from build123d import *

# Parameters (mm, degrees)
F1_DEPTH = 50
F3_DEPTH = 25
F4_R     = 9
F5_DEPTH = 25


with BuildPart() as f1:
    # F0 (on Front) → F1 (new body)
    with BuildSketch(Plane.XZ):
        Polygon((48.981464, 6), (-26.018536, 6), (-26.018536, 29), (-36.018536, 29), (-36.018536, -6), (33.685692, -6), (33.685692, -16.768231), (43.685692, -16.768231), (48.981464, -6), align=None)
    extrude(amount=F1_DEPTH)

    # F2 (on face) → F3 (cut)
    with BuildSketch(Plane.YZ.offset(-26.018536)):
        Polygon((-20.902064, 29), (-30.902064, 29), (-30.902064, 21), (-35.902064, 21), (-35.902064, 13), (-15.902064, 13), (-15.902064, 21), (-20.902064, 21), align=None)
    extrude(amount=-F3_DEPTH, mode=Mode.SUBTRACT)

    # F4 (on face) → F5 (cut)
    with BuildSketch(Plane.XY.offset(6)):
        with Locations((13.981464, -25)):
            Circle(F4_R)
    extrude(amount=-F5_DEPTH, mode=Mode.SUBTRACT)


solid = f1.part
Check sheet for the modelled part. Datum: model origin and axes. Units: mm. A direction names the side the tool comes from. Round coordinates to 2 decimals unless told otherwise and drop trailing zeros. Loops run counter-clockwise (first coordinate to the right, second up) from the corner with the lowest first, then second, coordinate; pieces in that order, holes last. Notation, with made-up numbers: M 14.25,-24 L 39.25,-24 A27 ccw 39.25,12 Z; hole C -30.5,67 d7. An arc over 180 degrees is marked long. One line per item, written item: value.
(1) Sectioned sample at A-A, the plane y = -25. Record the cut outline in (x, z), then the cut area to 3 significant figures.
Computed values:
outline: M -36.02,-6 L 4.98,-6 L 4.98,6 L -26.02,6 L -26.02,13 L -36.02,13 Z; M 22.98,-6 L 33.69,-6 L 33.69,-16.77 L 43.69,-16.77 L 48.98,-6 L 48.98,6 L 22.98,6 Z
area: 1,010 mm^2
(2) Sectioned sample at B-B, the plane z = 24. Record the cut outline in (x, y), then the cut area to 3 significant figures.
Computed values:
outline: M -36.02,-50 L -26.02,-50 L -26.02,-30.9 L -36.02,-30.9 Z; M -36.02,-20.9 L -26.02,-20.9 L -26.02,0 L -36.02,0 Z
area: 400 mm^2
(3) Sectioned sample at D-D, the plane x = 17. Record the cut outline in (y, z).
Computed values:
outline: M -50,-6 L -33.48,-6 L -33.48,6 L -50,6 Z; M -16.52,-6 L 0,-6 L 0,6 L -16.52,6 Z
(4) Sectioned sample at C-C, the plane z = -1.5. Record the cut outline in (x, y).
Computed values:
outline: M -36.02,-50 L 48.98,-50 L 48.98,0 L -36.02,0 Z; hole C 13.98,-25 d18
(5) Access from +Z, -Z, +X, -X, +Y, -Y to the whole of each face (thin tool, end or side, straight path). Record for faces 1 (the face through (-31, -35.902, 17)), 2 (the face through (-26.019, -25, 12)), 3 (the face through (-31, -30.902, 25)).
Computed values:
face 1: +X, -X
face 2: +Z, +X, +Y, -Y
face 3: +Z, +X, -X
(6) Thickness scan on line 1 (X direction, y = -3, z = 7.5); line 2 (Z direction, x = -22.5, y = -46); line 3 (Z direction, x = 42, y = -41). Record the ranges inside material, lowest first.
Computed values:
line 1: x = -36.02 to -26.02
line 2: z = -6 to 6
line 3: z = -16.77 to 6
(7) Release check for a two-part mould opening along Z. For faces 4 (the face through (48.981, -25, 0)), 5 (the face through (-31, -15.902, 17)), 6 (the face through (-31, -40, 29)) record: +Z half, -Z half, draft (parallel to the pull), parting line (faces both ways), or undercut.
Computed values:
face 4: draft
face 5: undercut
face 6: +Z half
(8) Depth check by flat-ended pin: pin 1 Ø1 at (x, y) = (38, -25) entering from +Z; pin 2 Ø3 at (x, y) = (15.5, -44) entering from -Z; pin 3 Ø18.5 at (y, z) = (-16.5, 18) entering from +X. Enter the tip coordinate at first touch or a pass-through.
Computed values:
pin 1: stops at z = 6
pin 2: stops at z = -6
pin 3: stops at x = -26.02
